Can you work these out from the model? Positions are in its coordinate system, mm. Face numbers are marked on the shaded views. A direction names the side the tool comes from. Round coordinates to 2 decimals unless told otherwise and drop trailing zeros. Loops run counter-clockwise (first coordinate to the right, second up) from the corner with the lowest first, then second, coordinate; pieces in that order, holes last.
(1) I want a section at C-C on x = 252. Write out the boundary of the cut face in (y, z).
(2) Will these pins go through, and if not, where does the flat tip stop? pin 1 Ø20.5 at (x, z) = (25.4, 152.4) entering from +Y; pin 2 Ø1.5 at (x, y) = (310.5, 619) entering from -Z; pin 3 Ø7.5 at (y, z) = (513.5, -18.5) entering from -X; pin 4 Ø7 at (x, z) = (403.5, -4) entering from -Y.
(3) I want a section at D-D on z = 127.5. Write out the boundary of the cut face in (x, y) (3 decimals), plus the area to 3 significant figures.
(4) Which directions (+Z, -Z, +X, -X, +Y, -Y) give clear straight access to the entire face, cutting with the end or side of a thin tool? Please do the marked faces 5 and 6.
(5) Thinking about a two-plate mould opening in Y: for the marked faces 1, 2, 3 and 4, which applies, released by +Y, released by -Y, zero draft, split by the parting line, or undercut?
(6) I want a section at B-B on y = 476.5. Write out the boundary of the cut face in (x, z).
(7) If I drill on line 1 along Y through (x, z) = (70, 72); line 2 along Z through (x, y) = (25.4, 2.75); line 3 along Z through (x, y) = (189.5, 559), over which ranges is the centre line in solid material (lowest first)?
(8) I want a section at A-A on z = 62. Write out the boundary of the cut face in (x, y), plus the area to 3 significant figures.
from build123d import *

# Parameters (mm, degrees)
F1_DEPTH = 177.8
F2_T     = -6.35
F3_R     = 6.35
F4_DEPTH = 1079.501
F5_W     = 6.35
F5_H     = 812.8
F6_DEPTH = 25.4
F8_R     = 10.16
F9_DEPTH = 1079.501


with BuildPart() as f1:
    # F0 (on Top) → F1 (new body)
    with BuildSketch(Plane.XY):
        Polygon((0, 1079.5), (0, 0), (101.6, 0), (406.4, 133.35), (406.4, 539.75), (406.4, 946.15), (101.6, 1079.5), align=None)
    extrude(amount=F1_DEPTH)

    # F2
    f2_openings = [f1.faces().sort_by_distance(p)[0] for p in [
        (192.825932, 539.75, 177.8),
        (0, 539.75, 88.9),
        (406.4, 539.75, 88.9),
    ]]
    offset(amount=F2_T, openings=f2_openings)

    # F3 (on face) → F4 (cut, through all)
    with BuildSketch(Plane.XZ):
        with Locations((25.4, 152.4)):
            Circle(F3_R)
    extrude(amount=-F4_DEPTH, mode=Mode.SUBTRACT)

    # F5 (on face) → F6 (join)
    with BuildSketch(Plane(origin=(0, 0, 0), x_dir=(1, 0, 0), z_dir=(0, 0, -1))):
        with Locations((403.225, -539.75)):
            Rectangle(F5_W, F5_H)
    extrude(amount=F6_DEPTH)

    # F8
    f8_edges = [f1.edges().sort_by_distance(p)[0] for p in [
        (403.225, 133.35, -25.4),
        (403.225, 946.15, -25.4),
    ]]
    fillet(f8_edges, radius=F8_R)

    # F7 (on Front) → F9 (cut, through all)
    with BuildSketch(Plane.XZ):
        Polygon((406.4, 101.6), (406.4, 177.8), (101.6, 177.8), align=None)
    extrude(amount=-F9_DEPTH, mode=Mode.SUBTRACT)


solid = f1.part
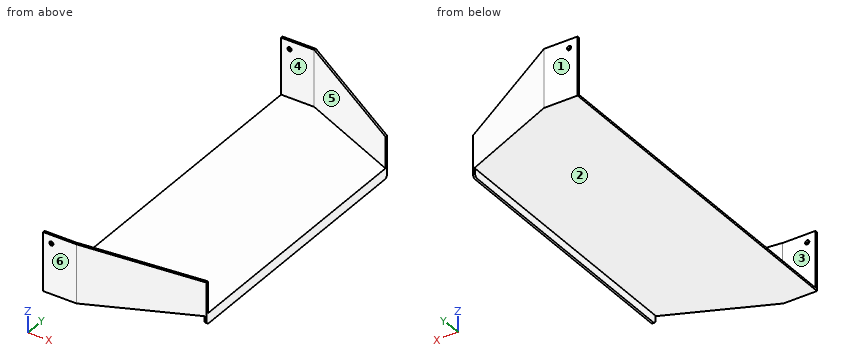
Filled sheet:
1. outline: (65.8, 0) - (1013.7, 0) - (1013.7, 140.2) - (1006.77, 140.2) - (1006.77, 6.35) - (72.73, 6.35) - (72.73, 140.2) - (65.8, 140.2) - close
2. pin 1: stops at y = 1079.5
2. pin 2: stops at z = 0
2. pin 3: stops at x = 400.05
2. pin 4: stops at y = 133.35
3. outline: (0, 0) - (101.6, 0) - (302.8, 88.025) - (302.8, 94.956) - (100.272, 6.35) - (0, 6.35) - close; (0, 1073.15) - (100.272, 1073.15) - (302.8, 984.544) - (302.8, 991.475) - (101.6, 1079.5) - (0, 1079.5) - close
3. area: 4,080 mm2
4. face 5: +Z, -X
4. face 6: +Z, -Z, +X, -X, -Y
5. face 1: released by +Y
5. face 2: zero draft
5. face 3: undercut
5. face 4: undercut
6. outline: (0, 0) - (400.05, 0) - (400.05, -25.4) - (406.4, -25.4) - (406.4, 6.35) - (0, 6.35) - close
7. line 1: y = 0 to 6.35, 1073.15 to 1079.5
7. line 2: z = 0 to 146.05, 158.75 to 177.8
7. line 3: z = 0 to 6.35
8. outline: (0, 0) - (101.6, 0) - (406.4, 133.35) - (406.4, 140.28) - (100.27, 6.35) - (0, 6.35) - close; (0, 1073.15) - (100.27, 1073.15) - (406.4, 939.22) - (406.4, 946.15) - (101.6, 1079.5) - (0, 1079.5) - close
8. area: 5,520 mm2
